from build123d import *

# Parameters (mm, degrees)
F0_W     = 120
F0_H     = 120
F0_R     = 42.5
F1_DEPTH = 260
F2_DEPTH = 130
F3_R     = 42.5
F5_DEPTH = 180
F4_R     = 42.5
F6_DEPTH = 180
F7_DEPTH = 20


with BuildPart() as f1:
    # F0 (on Top) → F1 (new body)
    with BuildSketch(Plane.XY):
        Rectangle(F0_W, F0_H)
        Circle(F0_R, mode=Mode.SUBTRACT)
    extrude(amount=F1_DEPTH)

    # F0 (on Top) → F2 (join)
    with BuildSketch(Plane.XY):
        with Locations((120, 0)):
            Rectangle(F0_W, F0_H)
        with Locations((0, -120)):
            Rectangle(F0_W, F0_H)
    extrude(amount=F2_DEPTH)

    # F3 (on face) → F5 (cut)
    with BuildSketch(Plane.XZ.offset(180)):
        with Locations((0, 65)):
            Circle(F3_R)
    extrude(amount=-F5_DEPTH, mode=Mode.SUBTRACT)

    # F4 (on face) → F6 (cut)
    with BuildSketch(Plane.YZ.offset(180)):
        with Locations((0, 65)):
            Circle(F4_R)
    extrude(amount=-F6_DEPTH, mode=Mode.SUBTRACT)

    # F0 (on Top) → F7 (join)
    with BuildSketch(Plane.XY):
        Circle(F0_R)
    extrude(amount=F7_DEPTH)


solid = f1.part
Can you work these out from the model? Positions are in its coordinate system, mm. A direction names the side the tool comes from. Give positions to 0.01 mm unless a question says otherwise; leave off trailing zeros. Loops run counter-clockwise (first coordinate to the right, second up) from the corner with the lowest first, then second, coordinate; pieces in that order, holes last. Notation, with made-up numbers: (-20.75, -2) - (2.25, -2) arc R26 ccw to (2.25, 13) - close; hole circle Ø3 at (65, 60). An arc over 180 degrees is marked (long way). One line per item, written item: value.
(1) If we section it at C-C, the plane z = 54.5: List the corners of the cut face in (x, y) for me, plus the area to 3 significant figures.
Verdict:
outline: (-60, -180) - (-41.18, -180) - (-41.18, -10.5) arc R42.5 cw to (10.5, 41.18) - (180, 41.18) - (180, 60) - (-60, 60) - close; (41.18, -180) - (60, -180) - (60, -60) - (180, -60) - (180, -41.18) - (41.18, -41.18) - close
area: 13,800 mm^2
(2) I'm going to push flat-ended pins straight in: pin 1 (6 mm diameter, centred on x = 34, y = -153, fed in from +Z); pin 2 (12 mm diameter, centred on x = 151, z = 137.5, fed in from +Y); pin 3 (2 mm diameter, centred on y = 16, z = 151.5, fed in from +X). Where does each tip first touch, or does it pass through?
Verdict:
pin 1: z = 130
pin 2: through
pin 3: x = 60
(3) If we section it at A-A, the plane x = 18: List the corners of the cut face in (y, z) for me, plus the area to 3 significant figures.
Verdict:
outline: (-180, 0) - (60, 0) - (60, 260) - (38.5, 260) - (38.5, 83) arc R42.5 cw to (38.5, 47) - (38.5, 20) - (-38.5, 20) - (-38.5, 26.5) - (-180, 26.5) - close; (-180, 103.5) - (-38.5, 103.5) - (-38.5, 260) - (-60, 260) - (-60, 130) - (-180, 130) - close
area: 17,300 mm^2
(4) I need wall thicknesses on line 1 along Y through (x, z) = (0, 121); line 2 along X through (y, z) = (0, 197); line 3 along X through (y, z) = (-49.5, 65). Which ranges of each line are inside material? Lowest first, please.
Verdict:
line 1: -180 to -42.5, 42.5 to 60
line 2: -60 to -42.5, 42.5 to 60
line 3: -60 to -42.5, 42.5 to 180
(5) On a 3-axis mill with a long thin cutter (end or side, diameter ignored), from which of +Z, -Z, +X, -X, +Y, -Y can I reach the whole of each face in a straight line? I mean faces 5 (the face through (119, -60, 64)), 6 (the face through (-42.46, -111.26, 66.87)), 7 (the face through (-1, -60, 194)), 8 (the face through (60, -1, 194)). Say none if no direction works.
Verdict:
face 5: +Z, -Z, +X, -Y
face 6: -Y
face 7: +Z, +X, -X, -Y
face 8: +Z, +X, +Y, -Y
(6) If we section it at D-D, the plane y = -47.5: List the corners of the cut face in (x, z) for me.
Verdict:
outline: (-60, 0) - (180, 0) - (180, 130) - (60, 130) - (60, 260) - (-60, 260) - close; hole circle Ø85 at (0, 65)
(7) If we section it at B-B, the plane y = -18: List the corners of the cut face in (x, z) for me, plus the area to 3 significant figures.
Verdict:
outline: (-60, 0) - (180, 0) - (180, 26.5) - (38.5, 26.5) - (38.5, 20) - (-38.5, 20) - (-38.5, 47) arc R42.5 cw to (-38.5, 83) - (-38.5, 260) - (-60, 260) - close; (38.5, 103.5) - (180, 103.5) - (180, 130) - (60, 130) - (60, 260) - (38.5, 260) - close
area: 17,300 mm^2
(8) If we mould it in two halves opening along Y, with no side actions, what happens to faces 1 (the face through (-1, 1, 20)), 2 (the face through (32, 60, 99)), 3 (the face through (111.26, 40.537, 77.766)), 4 (the face through (60, -121, 64))? For each: released by +Y, released by -Y, zero draft, split by the parting line, or undercut.
Verdict:
face 1: undercut
face 2: released by +Y
face 3: undercut
face 4: zero draft
